Part model, mm, in its own coordinate system. Face numbers are marked on the shaded views. A direction names the side the tool comes from. Round coordinates to 2 decimals unless told otherwise and drop trailing zeros. Write each loop counter-clockwise with the first axis right and the second up, starting at its lowest first coordinate (ties: lowest second). Pieces come first, ordered by that corner, then holes.
1) Saw through at D-D on y = 178. Write the cut outline in (x, z), and give its area (3 significant figures).
2) Saw through at A-A on x = -544. Write the cut outline in (y, z), and give its area (3 significant figures).
3) Flat gauge pin, fed straight in: pin 1 (10 mm diameter, centred on x = -554.5, y = 673, fed in from -Z). Where does the tip first touch, or does it go through?
4) Which spindle directions (+Z, -Z, +X, -X, +Y, -Y) get a long thin tool onto all of the face, cutting with end or side? Do the marked faces 1 and 2. Say none if no direction does.
5) Drill centre lines: L1, parallel to X at y = 473, z = 245; L2, parallel to Y at x = 412, z = 465; L3, parallel to Z at x = 763.5, y = -825. Where is each one in solid material? Low to high.
6) Saw through at B-B on z = 336. Write the cut outline in (x, y).
7) Pull direction X, two halves, no side cores. Call the marked faces 3, 4 and 5: +X half, -X half, draft (parallel to the pull), parting line (faces both ways), or undercut.
8) Saw through at C-C on z = 221. Write the cut outline in (x, y), and give its area (3 significant figures).
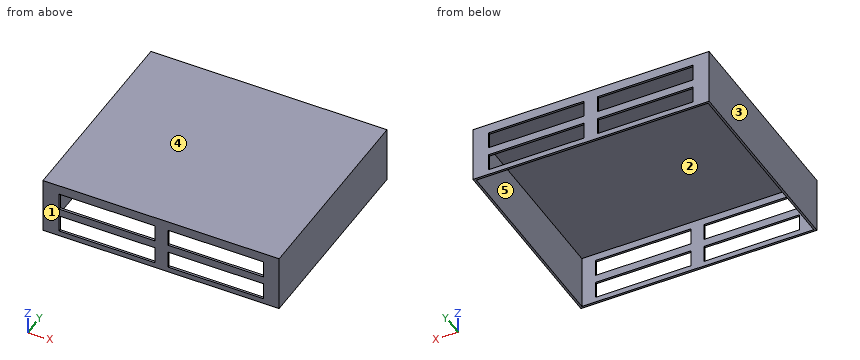
```python
from build123d import *

# Parameters (mm, degrees)
F0_W     = 2083
F0_H     = 1808
F1_DEPTH = 500
F2_T     = -19
F3_W     = 843.087125
F3_H     = 150.265902
F4_DEPTH = 19
F5_W     = 843.087125
F5_H     = 150.265902
F6_DEPTH = 19


with BuildPart() as f1:
    # F0 (on Top) → F1 (new body)
    with BuildSketch(Plane.XY):
        Rectangle(F0_W, F0_H)
    extrude(amount=F1_DEPTH)

    # F2
    f2_openings = [f1.faces().sort_by_distance(p)[0] for p in [
        (0, 0, 0),
    ]]
    offset(amount=F2_T, openings=f2_openings)

    # F3 (on face) → F4 (cut, through all)
    with BuildSketch(Plane.XZ.offset(904)):
        with Locations((-477.065479, 341.865197)):
            Rectangle(F3_W, F3_H)
        with Locations((482.93452, 341.865197)):
            Rectangle(F3_W, F3_H)
        with Locations((-477.065479, 121.865197)):
            Rectangle(F3_W, F3_H)
        with Locations((482.93452, 121.865197)):
            Rectangle(F3_W, F3_H)
    extrude(amount=-F4_DEPTH, mode=Mode.SUBTRACT)

    # F5 (on face) → F6 (cut, through all)
    with BuildSketch(Plane(origin=(0, 904, 0), x_dir=(-1, 0, 0), z_dir=(0, 1, 0))):
        with Locations((-482.93452, 341.865197)):
            Rectangle(F5_W, F5_H)
        with Locations((477.065479, 341.865197)):
            Rectangle(F5_W, F5_H)
        with Locations((-482.93452, 121.865197)):
            Rectangle(F5_W, F5_H)
        with Locations((477.065479, 121.865197)):
            Rectangle(F5_W, F5_H)
    extrude(amount=-F6_DEPTH, mode=Mode.SUBTRACT)


solid = f1.part
```
Completed:
1. outline: (-1041.5, 0) - (-1022.5, 0) - (-1022.5, 481) - (1022.5, 481) - (1022.5, 0) - (1041.5, 0) - (1041.5, 500) - (-1041.5, 500) - close
1. area: 57,900 mm2
2. outline: (-904, 0) - (-885, 0) - (-885, 46.73) - (-904, 46.73) - close; (-904, 197) - (-885, 197) - (-885, 266.73) - (-904, 266.73) - close; (-904, 417) - (-885, 417) - (-885, 481) - (885, 481) - (885, 417) - (904, 417) - (904, 500) - (-904, 500) - close; (885, 0) - (904, 0) - (904, 46.73) - (885, 46.73) - close; (885, 197) - (904, 197) - (904, 266.73) - (885, 266.73) - close
2. area: 41,200 mm2
3. pin 1: stops at z = 481
4. face 1: +Z, -Z, +X, -X, -Y
4. face 2: -Z
5. L1: x = -1041.5 to -1022.5, 1022.5 to 1041.5
5. L2: y = -904 to -885, 885 to 904
5. L3: z = 481 to 500
6. outline: (-1041.5, -904) - (-898.61, -904) - (-898.61, -885) - (-1022.5, -885) - (-1022.5, 885) - (-898.61, 885) - (-898.61, 904) - (-1041.5, 904) - close; (-55.52, -904) - (61.39, -904) - (61.39, -885) - (-55.52, -885) - close; (-55.52, 885) - (61.39, 885) - (61.39, 904) - (-55.52, 904) - close; (904.48, -904) - (1041.5, -904) - (1041.5, 904) - (904.48, 904) - (904.48, 885) - (1022.5, 885) - (1022.5, -885) - (904.48, -885) - close
7. face 3: -X half
7. face 4: draft
7. face 5: undercut
8. outline: (-1041.5, -904) - (1041.5, -904) - (1041.5, 904) - (-1041.5, 904) - close; hole (-1022.5, -885) - (1022.5, -885) - (1022.5, 885) - (-1022.5, 885) - close
8. area: 146,000 mm2
